Input: part model. Units: mm. Frame: model coordinates. A direction names the side the tool comes from. Round coordinates to 2 decimals unless told otherwise and drop trailing zeros. Order: outer loops, then holes, each group sorted by start corner. A loop starts at its lowest first (then second) coordinate and runs counter-clockwise, first axis right, second up.
Item 1: Cut plane B-B on z = 11. Output: boundary loops of the cut face in (x, y).
Item 2: Reachability of faces 5 (the cylindrical face through (7.273, 3.974, 11.914)), 6 (the cylindrical face through (0.36, 6.85, -7.14)) from +Z, -Z, +X, -X, +Y, -Y: full face, straight path, thin tool, end or side. Return the list, or none.
Item 3: Cut plane C-C on x = -5.16. Output: boundary loops of the cut face in (y, z), then the cut area to 3 significant figures.
Item 4: Cut plane A-A on y = 1.5. Output: boundary loops of the cut face in (x, z), then the cut area to 3 significant figures.
Item 5: Line query: L1, parallel to X at y = 4.25, z = 0; L2, parallel to Y at x = 0, z = -2.5; L3, parallel to Z at x = 18, y = 2.25. Output: solid intervals per line, ascending.
Item 6: Cut plane D-D on z = 0. Output: boundary loops of the cut face in (x, y).
Item 7: Mould query, pull axis Z, two halves, no side actions, for faces 1 (the flat face through (0, 4, 17.5)), 2 (the flat face through (6, 5.838, 4)), 3 (the flat face through (0, 4, -17.5)), 4 (the flat face through (22.5, 4, 0)). Classes: released by +Z, released by -Z, zero draft, split by the parting line, or undercut.
```python
from build123d import *

# Parameters (mm, degrees)
SKETCH1_W           = 45
SKETCH1_H           = 35
BOSS_EXTRUDE1_DEPTH = 7.838444594
SKETCH4_R           = 9
CUT_EXTRUDE3_DEPTH  = 2
SKETCH5_R           = 1.7
SKETCH5_R_2         = 3
CUT_EXTRUDE4_DEPTH  = 7.838444594


with BuildPart() as part:
    # Sketch1 → Boss-Extrude1 (new body)
    with BuildSketch(Plane(origin=(0, 0, 0), x_dir=(1, 0, 0), z_dir=(0, 1, 0))):
        Rectangle(SKETCH1_W, SKETCH1_H)
    extrude(amount=BOSS_EXTRUDE1_DEPTH)

    # Sketch4 → Cut-Extrude3 (cut)
    with BuildSketch(Plane(origin=(0, 7.838444594, 0), x_dir=(1, 0, 0), z_dir=(0, 1, 0))):
        with Locations(Location((5.84, 0, 0), (0, 0, 270))):
            Circle(SKETCH4_R)
    extrude(amount=-CUT_EXTRUDE3_DEPTH, mode=Mode.SUBTRACT)

    # Sketch5 → Cut-Extrude4 (cut)
    with BuildSketch(Plane(origin=(0, 7.838444594, 0), x_dir=(1, 0, 0), z_dir=(0, 1, 0))):
        with Locations(Location((5.84, 11, 0), (0, 0, 270))):
            Circle(SKETCH5_R)
        with Locations(Location((16.84, 0, 0), (0, 0, 270))):
            Circle(SKETCH5_R)
        with Locations(Location((5.84, -11, 0), (0, 0, 270))):
            Circle(SKETCH5_R)
        with Locations(Location((-5.16, 0, 0), (0, 0, 270))):
            Circle(SKETCH5_R)
        with Locations(Location((5.84, 0, 0), (0, 0, 270))):
            Circle(SKETCH5_R_2)
    extrude(amount=-CUT_EXTRUDE4_DEPTH, mode=Mode.SUBTRACT)


solid = part.part
```
From the geometry:
1. outline: (-22.5, 0) - (4.14, 0) - (4.14, 7.84) - (-22.5, 7.84) - close; (7.54, 0) - (22.5, 0) - (22.5, 7.84) - (7.54, 7.84) - close
2. face 5: +Y, -Y
2. face 6: +Y
3. outline: (0, -17.5) - (7.84, -17.5) - (7.84, -1.7) - (0, -1.7) - close; (0, 1.7) - (7.84, 1.7) - (7.84, 17.5) - (0, 17.5) - close
3. area: 248 mm2
4. outline: (-22.5, -17.5) - (22.5, -17.5) - (22.5, 17.5) - (-22.5, 17.5) - close; hole circle Ø3.4 at (-5.16, 0); hole circle Ø6 at (5.84, 0); hole circle Ø3.4 at (5.84, -11); hole circle Ø3.4 at (5.84, 11); hole circle Ø3.4 at (16.84, 0)
4. area: 1,510 mm2
5. L1: x = -22.5 to -6.86, -3.46 to 2.84, 8.84 to 15.14, 18.54 to 22.5
5. L2: y = 0 to 5.84
5. L3: z = -17.5 to -1.24, 1.24 to 17.5
6. outline: (-22.5, 0) - (-6.86, 0) - (-6.86, 7.84) - (-22.5, 7.84) - close; (-3.46, 0) - (2.84, 0) - (2.84, 5.84) - (-3.16, 5.84) - (-3.16, 7.84) - (-3.46, 7.84) - close; (8.84, 0) - (15.14, 0) - (15.14, 7.84) - (14.84, 7.84) - (14.84, 5.84) - (8.84, 5.84) - close; (18.54, 0) - (22.5, 0) - (22.5, 7.84) - (18.54, 7.84) - close
7. face 1: released by +Z
7. face 2: undercut
7. face 3: released by -Z
7. face 4: zero draft
